For this review, take the finished solid that the model builds, in its own axes (mm). A direction names the side the tool comes from. Round coordinates to 2 decimals unless told otherwise and drop trailing zeros. Order: outer loops, then holes, each group sorted by start corner. A loop starts at its lowest first (then second) coordinate and runs counter-clockwise, first axis right, second up. Notation, with made-up numbers: (42.5, 51) -> (79.5, 51) arc R12 ccw to (79.5, 66) -> close; hole circle Ø7 at (-40, 35.5). An arc over 180 degrees is marked (long way). Answer in a Markdown table with one row per item.
Autodesk Inventor part; units mm, degrees
ref_plane "YZ Plane" through (0, 0, 0) normal (1, 0, 0) x (0, 1, 0)
ref_plane "XZ Plane" through (0, 0, 0) normal (0, 1, 0) x (-1, 0, 0)
ref_plane "XY Plane" through (0, 0, 0) normal (0, 0, 1) x (1, 0, 0)
sketch "草图1" plane through (0, 0, 0) normal (0, 1, 0) x (-1, 0, 0)
  line L0 (0, 0) -> (-6, 0) construction
  line L1 (0, 3) -> (-6, 3)
  line L2 (-6, -3) -> (0, -3)
  arc A0 (0, -3) -> (0, 3) centre (0, 0) ccw
  arc A1 (-6, 3) -> (-6, -3) centre (-6, 0) ccw
  circle A2 centre (0, 0) radius 1.5
  circle A3 centre (-6, 0) radius 1.5
  point P0 (-3, 0)
  dimension "d0" = 6
  dimension "d1" = 3
  dimension "d2" = 3
  dimension "d3" = 1.5
extrude "拉伸1" add sketch "草图1" along normal blind 5
sketch "草图2" plane through (6, 0, -3) normal (0, 0, -1) x (-1, 0, 0)
  line L0 (0, 0) -> (6, 0)
  line L1 (6, 0) -> (6, 5)
  line L2 (0, 5) -> (6, 5)
  line L3 (0, 0) -> (0, 5)
  line L4 (0, 0) -> (6, 0)
  line L5 (6, 0) -> (6, 5)
  line L6 (6, 5) -> (0, 5)
  line L7 (0, 5) -> (0, 0)
  line L8 (0, 0) -> (6, 5) construction
  line L9 (6, 0) -> (0, 5) construction
  line L10 (0, 5) -> (6, 5)
  line L11 (6, 0) -> (6, 5)
  line L12 (0, 0) -> (6, 0)
  line L13 (0, 0) -> (0, 5)
  circle A0 centre (3, 2.5) radius 1.5
  dimension "d6" = 3
extrude "拉伸2" add sketch "草图2" along normal blind 5
properties part number "夹爪连接件"
Q1. Tool access review of faces 1 (the face through (0, 2, -5)), 2 (the face through (6, 2, -5)), 3 (the face through (3, 2, -3)), 4 (the face through (9, 2, 0)), 5 (the face through (-3, 2, 0)): name each direction out of +Z, -Z, +X, -X, +Y, -Y from which nothing blocks a thin tool from reaching the whole face with its end or side.
Answer key:
| item | result |
|---|---|
| face 1 | -Z, -X, +Y, -Y |
| face 2 | -Z, +X, +Y, -Y |
| face 3 | -Z |
| face 4 | +X, +Y, -Y |
| face 5 | -X, +Y, -Y |
Q2. Take a section at C-C, the plane x = 0.5. Write out the cut boundary in (y, z).
Answer key:
| item | result |
|---|---|
| outline | (0, -8) -> (5, -8) -> (5, -1.41) -> (0, -1.41) -> close; (0, 1.41) -> (5, 1.41) -> (5, 3) -> (0, 3) -> close |
Q3. Take a section at B-B, the plane y = 2.5. Write out the cut boundary in (x, z).
Answer key:
| item | result |
|---|---|
| outline | (0, -8) -> (1.5, -8) -> (1.5, -3) -> (4.5, -3) -> (4.5, -8) -> (6, -8) -> (6, -3) arc R3 ccw to (6, 3) -> (0, 3) arc R3 ccw to (0, -3) -> close; hole circle Ø3 at (0, 0); hole circle Ø3 at (6, 0) |
Q4. The part is to be moulded in two halves that separate along Y. For faces 6 (the face through (1.5, 2.46, -0.07)), 7 (the face through (3, 0, -2)), 8 (the face through (2.194, 1.235, -5.465)), say which applies: +Y half, -Y half, draft (parallel to the pull), parting line (faces both ways), or undercut.
Answer key:
| item | result |
|---|---|
| face 6 | draft |
| face 7 | -Y half |
| face 8 | undercut |
Q5. Take a section at A-A, the plane z = 0. Write out the cut boundary in (x, y).
Answer key:
| item | result |
|---|---|
| outline | (-3, 0) -> (-1.5, 0) -> (-1.5, 5) -> (-3, 5) -> close; (1.5, 0) -> (4.5, 0) -> (4.5, 5) -> (1.5, 5) -> close; (7.5, 0) -> (9, 0) -> (9, 5) -> (7.5, 5) -> close |
Q6. Take a section at D-D, the plane z = -4.25. Write out the cut boundary in (x, y).
Answer key:
| item | result |
|---|---|
| outline | (0, 0) -> (6, 0) -> (6, 5) -> (0, 5) -> close; hole circle Ø3 at (3, 2.5) |
Q7. To check wall thickness, follow probe 1 along Y at (x, z) = (3, -5.4); probe 2 along X at (y, z) = (2.4, -3.5); probe 3 along Z at (x, y) = (5, 3.55). State the ranges of each line that lie inside material, in increasing order.
Answer key:
| item | result |
|---|---|
| probe 1 | y = 0 to 1, 4 to 5 |
| probe 2 | x = 0 to 1.5, 4.5 to 6 |
| probe 3 | z = -8 to -1.12, 1.12 to 3 |
Q8. Clearance check with flat-ended pins moving along their axes: pin 1 Ø1.8 at (x, z) = (0, 0) entering from +Y; pin 2 Ø1.5 at (x, y) = (3, 2) entering from -Z; pin 3 Ø1.5 at (y, z) = (2, -5) entering from -X. State where each tip first meets the part, or that it passes through.
Answer key:
| item | result |
|---|---|
| pin 1 | passes through |
| pin 2 | stops at z = -3 |
| pin 3 | stops at x = 0 |
